Work out the finished part from the listing and answer in its coordinate system (mm). Face numbers are marked on the shaded views. A direction names the side the tool comes from. Coordinates: 2 decimals unless noted, no trailing zeros. Loops run counter-clockwise (first coordinate to the right, second up) from the corner with the lowest first, then second, coordinate; pieces in that order, holes last. Notation, with made-up numbers: (37.25, 42.5) - (63.25, 42.5) arc R11 cw to (63.25, 50.5) - close; hole circle Ø4 at (5, 82.25). An arc over 180 degrees is marked (long way). Write each question's results on one line, items separated by ' | '. Start each with the question number.
Item 1: Section D-D, the plane x = 3 is taken. Write down the section's boundary in (y, z), plus the area to 3 significant figures.
Item 2: Section A-A, the plane z = 11 is taken. Write down the section's boundary in (x, y).
Item 3: A tool of negligible diameter and unlimited length cuts with its end or side. For the marked faces 1 and 2, from which of +Z, -Z, +X, -X, +Y, -Y can it reach the whole face along a straight path? Write none if from no direction.
Item 4: Each of these flat-tipped pins is pushed along its axis until it touches: pin 1 Ø3 at (y, z) = (-15, 8.5) entering from -X; pin 2 Ø6.5 at (x, y) = (-14.2, -6.88) entering from -Z. Where does it stop, or does it pass through?
Item 5: Section C-C, the plane y = -7 is taken. Write down the section's boundary in (x, z).
Item 6: Consider probe 1 along Z at (x, y) = (18, 14); probe 2 along X at (y, z) = (12, 5.75); probe 3 along Z at (x, y) = (5.5, -12). Determine where each line is inside the solid, lowest interval first. Write a range as [from, to].
Item 7: Section B-B, the plane x = 7 is taken. Write down the section's boundary in (y, z).
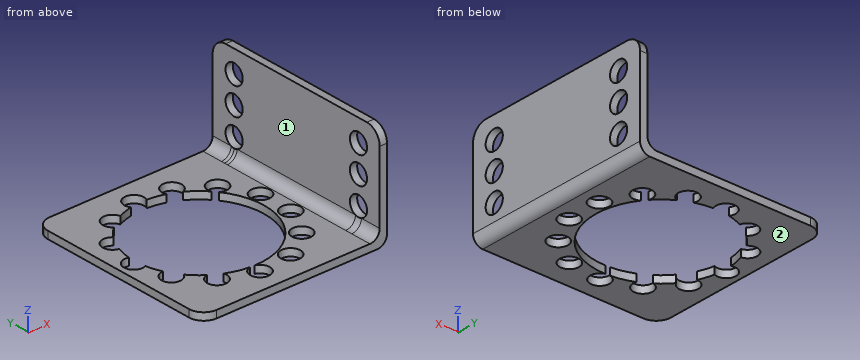
from build123d import *

# Parameters (mm, degrees)
SKETCH1_W               = 38
SKETCH1_H               = 38.950729927
SKETCH1_R               = 13.294995111
BOSS_EXTRUDE1_DEPTH     = 1.5
SKETCH4_W               = 19.5
SKETCH4_H               = 38.950729927
BOSS_EXTRUDE2_DEPTH     = 1.5
CUT_EXTRUDE2_DEPTH      = 35.383862494
CUT_EXTRUDE2_DEPTH_BACK = 35.383862494
SKETCH5_R               = 2
FILLET2_R               = 3
FILLET6_R               = 2
SKETCH6_R               = 1.98665291
CUT_EXTRUDE5_DEPTH      = 1.5


with BuildPart() as part:
    # Sketch1 → Boss-Extrude1 (new body)
    with BuildSketch(Plane.XY):
        with Locations((0, 0.024635036)):
            Rectangle(SKETCH1_W, SKETCH1_H)
        with Locations((-2, 0.5)):
            Circle(SKETCH1_R, mode=Mode.SUBTRACT)
    extrude(amount=BOSS_EXTRUDE1_DEPTH)

    # Sketch4 → Boss-Extrude2 (add)
    with BuildSketch(Plane(origin=(19, 0, 0), x_dir=(0, 0, -1), z_dir=(1, 0, 0))):
        with Locations((-11.25, 0.024635036)):
            Rectangle(SKETCH4_W, SKETCH4_H)
    extrude(amount=-BOSS_EXTRUDE2_DEPTH)

    # Sketch5 → Cut-Extrude2 (cut, two sides: drawn at the far end of the back side and taken through both)
    with BuildSketch(Plane(origin=(0, 0, 0), x_dir=(0, 0, -1), z_dir=(1, 0, 0)).offset(-CUT_EXTRUDE2_DEPTH_BACK)):
        with Locations((-5.375668666, 14.5)):
            Circle(SKETCH5_R)
        with Locations((-11, 14.5)):
            Circle(SKETCH5_R)
        with Locations((-16.492234483, 14.5)):
            Circle(SKETCH5_R)
        with Locations(Location((-16.492234483, -14.5, 0), (0, 0, 270))):
            Circle(SKETCH5_R)
        with Locations(Location((-11, -14.5, 0), (0, 0, 270))):
            Circle(SKETCH5_R)
        with Locations(Location((-5.375668666, -14.5, 0), (0, 0, 270))):
            Circle(SKETCH5_R)
    extrude(amount=CUT_EXTRUDE2_DEPTH + CUT_EXTRUDE2_DEPTH_BACK, mode=Mode.SUBTRACT)

    # Fillet2
    fillet2_edges = [part.edges().sort_by_distance(p)[0] for p in [
        (18.25, -19.450729927, 21),
        (18.25, 19.5, 21),
        (-19, -19.450729927, 0.75),
        (-19, 19.5, 0.75),
    ]]
    fillet(fillet2_edges, radius=FILLET2_R)

    # Fillet6
    fillet6_edges = [part.edges().sort_by_distance(p)[0] for p in [
        (19, 0.024635036, 0),
        (17.5, 0.024635036, 1.5),
    ]]
    fillet(fillet6_edges, radius=FILLET6_R)

    # Sketch6 → Cut-Extrude5 (cut)
    with BuildSketch(Plane.XY):
        with Locations((-15.899992969, 0)):
            Circle(SKETCH6_R)
        with Locations((-14.204742149, 6.877902946)):
            Circle(SKETCH6_R)
        with Locations((-9.507351221, 12.180161215)):
            Circle(SKETCH6_R)
        with Locations((-2.883935837, 14.692091337)):
            Circle(SKETCH6_R)
        with Locations((4.148159359, 13.838240392)):
            Circle(SKETCH6_R)
        with Locations((9.977966104, 9.814215342)):
            Circle(SKETCH6_R)
        with Locations((13.269945929, 3.541871831)):
            Circle(SKETCH6_R)
        with Locations((13.269945929, -3.541871831)):
            Circle(SKETCH6_R)
        with Locations((9.977966104, -9.814215342)):
            Circle(SKETCH6_R)
        with Locations((4.148159359, -13.838240392)):
            Circle(SKETCH6_R)
        with Locations((-2.883935837, -14.692091337)):
            Circle(SKETCH6_R)
        with Locations((-9.507351221, -12.180161215)):
            Circle(SKETCH6_R)
        with Locations((-14.204742149, -6.877902946)):
            Circle(SKETCH6_R)
    extrude(amount=CUT_EXTRUDE5_DEPTH, mode=Mode.SUBTRACT)


solid = part.part
Answer key:
1) outline: (-19.45, 0) - (-15.46, 0) - (-15.46, 1.5) - (-19.45, 1.5) - close; (-12.22, 0) - (-11.82, 0) - (-11.82, 1.5) - (-12.22, 1.5) - close; (15.46, 0) - (19.5, 0) - (19.5, 1.5) - (15.46, 1.5) - close | area: 12.6 mm^2
2) outline: (17.5, -19.45) - (19, -19.45) - (19, -16.5) - (17.5, -16.5) - close; (17.5, -12.5) - (19, -12.5) - (19, 12.5) - (17.5, 12.5) - close; (17.5, 16.5) - (19, 16.5) - (19, 19.5) - (17.5, 19.5) - close
3) face 1: +Z, -X, +Y, -Y | face 2: -Z, +X, -X, +Y, -Y
4) pin 1: stops at x = 17.5 | pin 2: stops at z = 0
5) outline: (-19, 0) - (-16.19, 0) - (-16.19, 1.5) - (-19, 1.5) - close; (8.98, 0) - (17, 0) arc R2 ccw to (19, 2) - (19, 21) - (17.5, 21) - (17.5, 3.5) arc R2 cw to (15.5, 1.5) - (8.98, 1.5) - close
6) probe 1: z = [0.27, 3.44], [7.31, 9.06], [12.94, 14.56], [18.43, 21] | probe 2: x = [17.5, 19] | probe 3: z = [0, 1.5]
7) outline: (-19.45, 0) - (-9.29, 0) - (-9.29, 1.5) - (-19.45, 1.5) - close; (10.29, 0) - (19.5, 0) - (19.5, 1.5) - (10.29, 1.5) - close
